Read the model definition and answer for the solid it produces. Units are mm, in the model's axes. Face numbers are marked on the shaded views. A direction names the side the tool comes from. Give positions to 0.01 mm unless a question says otherwise; leave off trailing zeros. Write each loop counter-clockwise with the first axis right and the second up, starting at its lowest first coordinate (ties: lowest second). Pieces come first, ordered by that corner, then holes. Notation, with made-up numbers: (75, 19) - (101, 19) arc R29 ccw to (101, 44) - close; hole circle Ø11 at (-11, 69). An arc over 180 degrees is marked (long way). Answer as a JSON object with one key per item and string values. Group by question number.
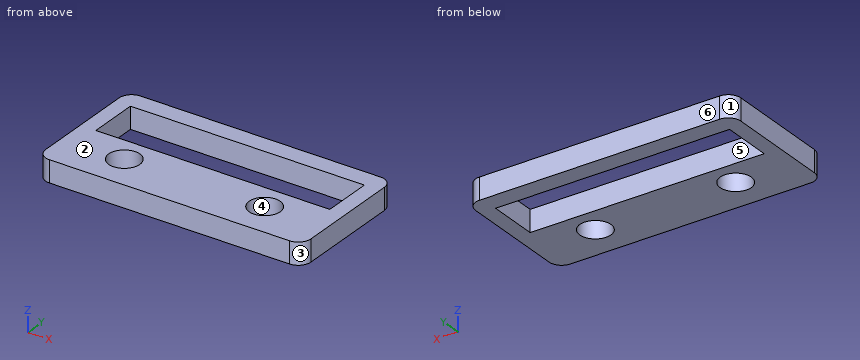
```python
from build123d import *

# Parameters (mm, degrees)
BOSS_EXTRUDE1_DEPTH = 7
SKETCH2_W           = 75
SKETCH2_H           = 16
CUT_EXTRUDE1_DEPTH  = 7
SKETCH3_R           = 5
CUT_EXTRUDE2_DEPTH  = 7


with BuildPart() as part:
    # Sketch1 → Boss-Extrude1 (new body)
    with BuildSketch(Plane.XY):
        with BuildLine():
            Line((-29.304093567, 27.587719298), (47.695906433, 27.587719298))
            ThreePointArc((47.695906433, 27.587719298), (50.524333557, 26.416146423), (51.695906433, 23.587719298))
            Line((51.695906433, 23.587719298), (51.695906433, -10.412280702))
            ThreePointArc((51.695906433, -10.412280702), (50.524333557, -13.240707827), (47.695906433, -14.412280702))
            Line((47.695906433, -14.412280702), (-29.304093567, -14.412280702))
            ThreePointArc((-29.304093567, -14.412280702), (-32.132520692, -13.240707827), (-33.304093567, -10.412280702))
            Line((-33.304093567, -10.412280702), (-33.304093567, 23.587719298))
            ThreePointArc((-33.304093567, 23.587719298), (-32.132520692, 26.416146423), (-29.304093567, 27.587719298))
        make_face()
    extrude(amount=BOSS_EXTRUDE1_DEPTH)

    # Sketch2 → Cut-Extrude1 (cut)
    with BuildSketch(Plane.XY.offset(7)):
        with Locations((9.195906433, 13.587719298)):
            Rectangle(SKETCH2_W, SKETCH2_H)
    extrude(amount=-CUT_EXTRUDE1_DEPTH, mode=Mode.SUBTRACT)

    # Sketch3 → Cut-Extrude2 (cut)
    with BuildSketch(Plane.XY.offset(7)):
        with Locations((31.695906433, -2.912280702)):
            Circle(SKETCH3_R)
        with Locations((-13.304093567, -2.912280702)):
            Circle(SKETCH3_R)
    extrude(amount=-CUT_EXTRUDE2_DEPTH, mode=Mode.SUBTRACT)


solid = part.part
```
1) Find section C-C, the plane y = -6.5. Write down the section's boundary in (x, z), and give its area (3 significant figures).
2) Find section D-D, the plane x = 34. Write down the section's boundary in (y, z), and give its area (3 significant figures).
3) Flat-ended cylindrical pins translate along their axes: pin 1 Ø1 at (x, y) = (-8, 6.5) entering from +Z; pin 2 Ø11.5 at (x, y) = (31.7, -2.91) entering from -Z. Find the tip coordinate at first contact, or state that the pin passes through.
4) For a pull along Y with two mould halves and no side action, classify the marked faces 1, 2, 3 and 4 as released by +Y, released by -Y, zero draft, split by the parting line, or undercut.
5) Which of the six approach directions +Z, -Z, +X, -X, +Y, -Y give full straight-line access (tool end or side, diameter ignored) to the marked faces 5 and 6?
6) Find section B-B, the plane x = 7.5. Write down the section's boundary in (y, z).
7) Find section A-A, the plane y = 17. Write down the section's boundary in (x, z), and give its area (3 significant figures).
8) Find the intervals of material crossed by line 1 (Y direction, x = 22, z = 4); line 2 (X direction, y = -6, z = 5); line 3 (X direction, y = -3.5, z = 1.75), in increasing order. Write a range as [from, to].
Values follow:
{
 "1": {"outline": "(-33.3, 0) - (-16.79, 0) - (-16.79, 7) - (-33.3, 7) - close; (-9.82, 0) - (28.21, 0) - (28.21, 7) - (-9.82, 7) - close; (35.18, 0) - (51.7, 0) - (51.7, 7) - (35.18, 7) - close", "area": "497 mm2"},
 "2": {"outline": "(-14.41, 0) - (-7.35, 0) - (-7.35, 7) - (-14.41, 7) - close; (1.53, 0) - (5.59, 0) - (5.59, 7) - (1.53, 7) - close; (21.59, 0) - (27.59, 0) - (27.59, 7) - (21.59, 7) - close", "area": "120 mm2"},
 "3": {"pin 1": "passes through", "pin 2": "stops at z = 0"},
 "4": {"face 1": "released by +Y", "face 2": "zero draft", "face 3": "released by -Y", "face 4": "undercut"},
 "5": {"face 5": "+Z, -Z", "face 6": "+Z, -Z, +X, -X, +Y"},
 "6": {"outline": "(-14.41, 0) - (5.59, 0) - (5.59, 7) - (-14.41, 7) - close; (21.59, 0) - (27.59, 0) - (27.59, 7) - (21.59, 7) - close"},
 "7": {"outline": "(-33.3, 0) - (-28.3, 0) - (-28.3, 7) - (-33.3, 7) - close; (46.7, 0) - (51.7, 0) - (51.7, 7) - (46.7, 7) - close", "area": "70.0 mm2"},
 "8": {"line 1": "y = [-14.41, 5.59], [21.59, 27.59]", "line 2": "x = [-33.3, -17.24], [-9.37, 27.76], [35.63, 51.7]", "line 3": "x = [-33.3, -18.27], [-8.34, 26.73], [36.66, 51.7]"}
}
